Study the drawing (mm; zero at the part's minimum x, y, z) and answer. Give positions to 0.01 mm unless a question says otherwise; leave off trailing zeros. Order: outer loops, then holes, each group sorted by start corner. A loop starts at its lowest first (then second) coordinate and runs counter-clockwise, first axis right, second up. Notation, with made-up numbers: (70, -26.75) -> (100, -26.75) arc R15 ccw to (100, -1.75) -> close; hole circle Ø1 at (-19.75, 39.25). An arc over 180 degrees is marked (long way). Answer as CSV lines item,"result". Start each with the question number.
1. For a pull along Y with two mould halves and no side action, classify the marked faces 1, 2, 3 and 4 as released by +Y, released by -Y, zero draft, split by the parting line, or undercut.
2. A cutting plane is placed at B-B (y = 9). Give the vertices of the cut face in (x, z).
3. A cutting plane is placed at D-D (z = 2.75). Give the vertices of the cut face in (x, y), then the cut area to 3 significant figures.
4. A cutting plane is placed at C-C (y = 17). Give the vertices of the cut face in (x, z).
5. A cutting plane is placed at A-A (x = 27.5). Give the vertices of the cut face in (y, z).
6. Find the intervals of material crossed by L1, parallel to X at y = 3, z = 6.25; L2, parallel to Y at x = 23, z = 1 (1 decimal); L3, parallel to Y at x = 36.5, z = 8.5 (1 decimal), in increasing order.
7. Flat-ended cylindrical pins translate along their axes: pin 1 (2 mm diameter, centred on x = 49.75, z = 6.35, fed in from +Y); pin 2 (4 mm diameter, centred on x = 5.25, z = 6.35, fed in from +Y) (1 decimal). Find the tip coordinate at first contact, or state that the pin passes through.
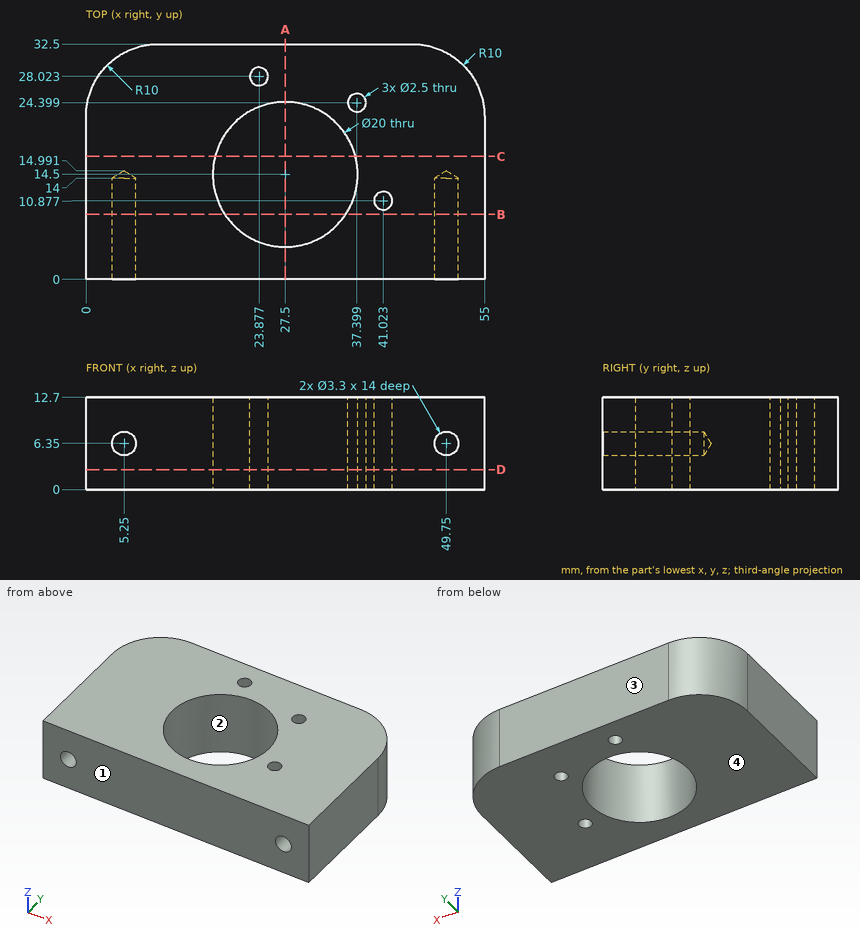
Answer sheet:
1,face 1,"released by -Y"
1,face 2,"undercut"
1,face 3,"released by +Y"
1,face 4,"zero draft"
2,outline,"(0, 0) -> (19.15, 0) -> (19.15, 12.7) -> (0, 12.7) -> close; (35.85, 0) -> (55, 0) -> (55, 12.7) -> (35.85, 12.7) -> close; hole circle Ø3.3 at (5.25, 6.35); hole circle Ø3.3 at (49.75, 6.35)"
3,outline,"(0, 0) -> (55, 0) -> (55, 22.5) arc R10 ccw to (45, 32.5) -> (10, 32.5) arc R10 ccw to (0, 22.5) -> close; hole circle Ø20 at (27.5, 14.5); hole circle Ø2.5 at (23.88, 28.02); hole circle Ø2.5 at (37.4, 24.4); hole circle Ø2.5 at (41.02, 10.88)"
3,area,"1,420 mm^2"
4,outline,"(0, 0) -> (17.82, 0) -> (17.82, 12.7) -> (0, 12.7) -> close; (37.18, 0) -> (55, 0) -> (55, 12.7) -> (37.18, 12.7) -> close"
5,outline,"(0, 0) -> (4.5, 0) -> (4.5, 12.7) -> (0, 12.7) -> close; (24.5, 0) -> (32.5, 0) -> (32.5, 12.7) -> (24.5, 12.7) -> close"
6,L1,"x = 0 to 3.6, 6.9 to 48.1, 51.4 to 55"
6,L2,"y = 0 to 5.6, 23.4 to 27.1, 28.9 to 32.5"
6,L3,"y = 0 to 10.1, 18.9 to 23.5, 25.3 to 32.5"
7,pin 1,"stops at y = 31.77"
7,pin 2,"stops at y = 32.1"
